Could you check a few things on this drawing? It's one solid part, dimensions in mm from its lowest x, y, z. A direction names the side the tool comes from. Coordinates: 2 decimals unless noted, no trailing zeros. Order: outer loops, then holes, each group sorted by start corner. A loop starts at its lowest first (then second) coordinate and runs counter-clockwise, first axis right, second up.
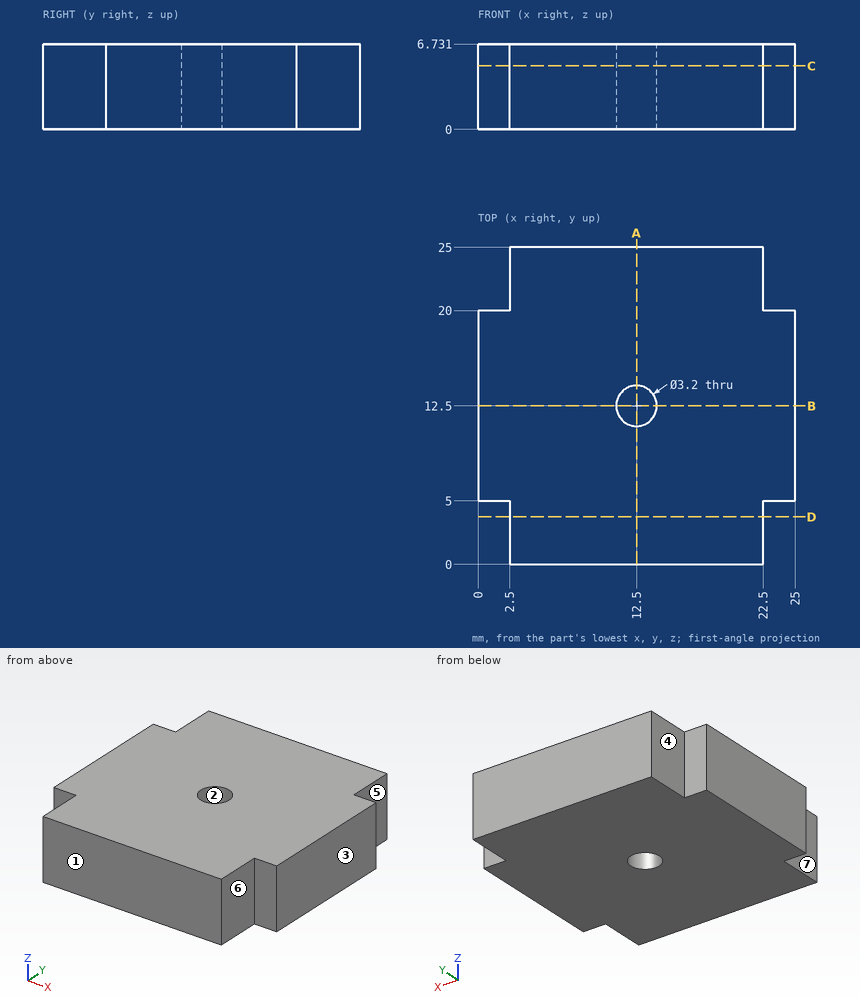
1. On a 3-axis mill with a long thin cutter (end or side, diameter ignored), from which of +Z, -Z, +X, -X, +Y, -Y can I reach the whole of each face in a straight line? I mean the marked faces 4, 5, 6 and 7. Say none if no direction works.
Completed:
face 4: +Z, -Z, -X, +Y
face 5: +Z, -Z, +X, +Y
face 6: +Z, -Z, +X, -Y
face 7: +Z, -Z, -X, -Y
2. Thinking about a two-plate mould opening in Y: for the marked faces 1, 2 and 3, which applies, pulls with the +Y half, pulls with the -Y half, needs draft (parallel to the pull), parting line crosses it, or undercut?
Completed:
face 1: pulls with the -Y half
face 2: undercut
face 3: needs draft
3. Imagine slicing it at A-A on x = 12.5. Please give me the cut outline in (y, z), then the cut area to 3 significant figures.
Completed:
outline: (0, 0) - (10.9, 0) - (10.9, 6.73) - (0, 6.73) - close; (14.1, 0) - (25, 0) - (25, 6.73) - (14.1, 6.73) - close
area: 147 mm2
4. Imagine slicing it at C-C on z = 5. Please give me the cut outline in (x, y), then the cut area to 3 significant figures.
Completed:
outline: (0, 5) - (2.5, 5) - (2.5, 0) - (22.5, 0) - (22.5, 5) - (25, 5) - (25, 20) - (22.5, 20) - (22.5, 25) - (2.5, 25) - (2.5, 20) - (0, 20) - close; hole circle Ø3.2 at (12.5, 12.5)
area: 567 mm2
5. I'm going to push flat-ended pins straight in: pin 1 (4 mm diameter, centred on y = 1.5, z = 3.5, fed in from -X); pin 2 (1.5 mm diameter, centred on y = 21.5, z = 3, fed in from +X); pin 3 (1.2 mm diameter, centred on x = 1, z = 3, fed in from -Y). Where does each tip first touch, or does it pass through?
Completed:
pin 1: stops at x = 2.5
pin 2: stops at x = 22.5
pin 3: stops at y = 5
6. Please list where these lines run through material, in increasing order: probe 1 along Y at (x, z) = (12.5, 3); probe 2 along Y at (x, z) = (2.25, 5); probe 3 along X at (y, z) = (12.25, 1.75).
Completed:
probe 1: y = 0 to 10.9, 14.1 to 25
probe 2: y = 5 to 20
probe 3: x = 0 to 10.92, 14.08 to 25
7. Imagine slicing it at D-D on y = 3.75. Please give me the cut outline in (x, z).
Completed:
outline: (2.5, 0) - (22.5, 0) - (22.5, 6.73) - (2.5, 6.73) - close
